Input: part model. Units: mm. Frame: model coordinates. Face numbers are marked on the shaded views. A direction names the side the tool comes from. Give positions to 0.01 mm unless a question says otherwise; leave off trailing zeros. Order: outer loops, then holes, each group sorted by start corner. A loop starts at its lowest first (then second) coordinate and runs counter-clockwise, first axis right, second up. Notation, with made-up numbers: (-3, 29.25) - (22, 29.25) arc R26 ccw to (22, 67.25) - close; hole circle Ø3 at (9, 52). An arc over 180 degrees is marked (long way). Use a Markdown table: item, result.
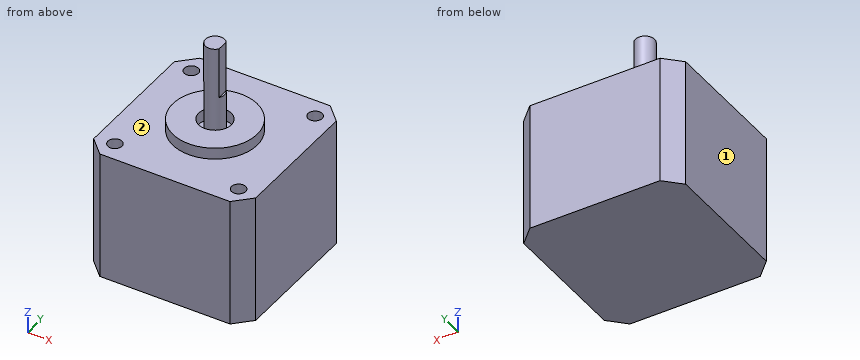
from build123d import *

# Parameters (mm, degrees)
F2_DEPTH      = 33.7
F3_R          = 11
F4_DEPTH      = 3
F5_R          = 4.25
F5_R_2        = 2.5
F6_DEPTH      = 3.1
F7_DEPTH      = 21
F7_DEPTH_BACK = 25.4
F9_DEPTH      = 13.4
F10_R         = 1.85
F11_DEPTH     = 4.75


with BuildPart() as f2:
    # F1 (on face) → F2 (new body)
    with BuildSketch(Plane.XY):
        Polygon((8.1, -21.15), (8.1, -18.0250372231), (-8.1, -18.0250372231), (-8.1, -21.15), (0, -21.15), align=None)
        Polygon((-8.1, -18.0250372231), (8.1, -18.0250372231), (8.1, -21.15), (17, -21.15), (21.15, -17), (21.15, 0), (21.15, 17), (17, 21.15), (0, 21.15), (-17, 21.15), (-21.15, 17), (-21.15, 0), (-21.15, -17), (-17, -21.15), (-8.1, -21.15), align=None)
    extrude(amount=F2_DEPTH)

    # F3 (on face) → F4 (join)
    with BuildSketch(Plane.XY.offset(33.7)):
        Circle(F3_R)
    extrude(amount=F4_DEPTH)

    # F5 (on face) → F6 (cut)
    with BuildSketch(Plane.XY.offset(36.7)):
        Circle(F5_R)
        Circle(F5_R_2, mode=Mode.SUBTRACT)
        Circle(F5_R_2)
    extrude(amount=-F6_DEPTH, mode=Mode.SUBTRACT)

    # F5 (on face) → F7 (join, two sides)
    with BuildSketch(Plane.XY.offset(36.7)) as f7_sk:
        Circle(F5_R_2)
    extrude(amount=F7_DEPTH)
    extrude(f7_sk.sketch, amount=-F7_DEPTH_BACK)

    # F8 (on face) → F9 (cut)
    with BuildSketch(Plane.XY.offset(57.7)):
        with BuildLine():
            Line((2, 1.5), (2, 0))
            Line((2, 0), (2, -1.5))
            ThreePointArc((2, -1.5), (2.3717082451, -0.790569415), (2.5, 0))
            ThreePointArc((2.5, 0), (2.3717082451, 0.790569415), (2, 1.5))
        make_face()
    extrude(amount=-F9_DEPTH, mode=Mode.SUBTRACT)

    # F10 (on face) → F11 (cut)
    with BuildSketch(Plane.XY.offset(33.7)):
        with Locations((-16.15, 16.1278136075)):
            Circle(F10_R)
        with Locations((16.15, 16.1278136075)):
            Circle(F10_R)
        with Locations((16.15, -16.1278136075)):
            Circle(F10_R)
        with Locations((-16.15, -16.1278136075)):
            Circle(F10_R)
    extrude(amount=-F11_DEPTH, mode=Mode.SUBTRACT)


solid = f2.part
1. Section query B-B (x = 16.15). Return loops of the section in (y, z), then the cut area to 3 significant figures.
Response:
| item | result |
|---|---|
| outline | (-21.15, 0) - (21.15, 0) - (21.15, 33.7) - (17.98, 33.7) - (17.98, 28.95) - (14.28, 28.95) - (14.28, 33.7) - (-14.28, 33.7) - (-14.28, 28.95) - (-17.98, 28.95) - (-17.98, 33.7) - (-21.15, 33.7) - close |
| area | 1,390 mm^2 |
2. Section query A-A (z = 35). Return loops of the section in (x, y), then the cut area to 3 significant figures.
Response:
| item | result |
|---|---|
| outline | circle Ø22 at (0, 0); circle Ø5 at (0, 0); hole circle Ø8.5 at (0, 0) |
| area | 343 mm^2 |
3. Pin query (flat end, axial travel): pin 1 (1.1 mm diameter, centred on x = -17, y = 16, fed in from +Z); pin 2 (3 mm diameter, centred on x = 17, y = -16.5, fed in from +Z); pin 3 (3.5 mm diameter, centred on y = 0.5, z = 52.5, fed in from +X). Return the tip coordinate at first contact, or that it passes through.
Response:
| item | result |
|---|---|
| pin 1 | stops at z = 28.95 |
| pin 2 | stops at z = 33.7 |
| pin 3 | stops at x = 2 |
4. Section query D-D (z = 6). Return loops of the section in (x, y).
Response:
| item | result |
|---|---|
| outline | (-21.15, -17) - (-17, -21.15) - (17, -21.15) - (21.15, -17) - (21.15, 17) - (17, 21.15) - (-17, 21.15) - (-21.15, 17) - close |
5. Section query C-C (y = 0). Return loops of the section in (x, z), then the cut area to 3 significant figures.
Response:
| item | result |
|---|---|
| outline | (-21.15, 0) - (21.15, 0) - (21.15, 33.7) - (11, 33.7) - (11, 36.7) - (4.25, 36.7) - (4.25, 33.6) - (2.5, 33.6) - (2.5, 44.3) - (2, 44.3) - (2, 57.7) - (-2.5, 57.7) - (-2.5, 33.6) - (-4.25, 33.6) - (-4.25, 36.7) - (-11, 36.7) - (-11, 33.7) - (-21.15, 33.7) - close |
| area | 1,580 mm^2 |
6. Material intervals for line 1 along Y through (x, z) = (16, 30); line 2 along Y through (x, z) = (0, 34); line 3 along Z through (x, y) = (18, -10), sorted ascending.
Response:
| item | result |
|---|---|
| line 1 | y = -21.15 to -17.97, -14.28 to 14.28, 17.97 to 21.15 |
| line 2 | y = -11 to -4.25, -2.5 to 2.5, 4.25 to 11 |
| line 3 | z = 0 to 33.7 |
7. Set-up query: the marked faces 1 and 2. Return all of +Z, -Z, +X, -X, +Y, -Y with unobstructed straight access to the full face (end or side cutting, diameter ignored); none if empty.
Response:
| item | result |
|---|---|
| face 1 | +Z, -Z, -X, +Y, -Y |
| face 2 | +Z |
